The drawing under review shows one solid part. Ordinate dimensions are in mm from its lowest x, y, z. A direction names the side the tool comes from. Coordinates: 2 decimals unless noted, no trailing zeros. Write each loop counter-clockwise with the first axis right and the second up, starting at its lowest first coordinate (ties: lowest second). Pieces come first, ordered by that corner, then holes. Notation, with made-up numbers: (55.25, -1) - (114.25, -1) arc R21 cw to (114.25, 37) - close; hole circle Ø5 at (20, -20). An arc over 180 degrees is marked (long way). Put each result on its own line as item: value. Start each with the question number.
Item 1: Consider section B-B on y = 449. Give the boundary of the cut face in (x, z) (3 decimals).
Item 2: Machinability: for the marked faces 5, 6 and 7, which of the approach directions +Z, -Z, +X, -X, +Y, -Y give a long, thin tool a straight path to every point of the face, cutting with its end or side? Answer none if there is none.
Item 3: Consider section A-A on x = 92.5. Give the boundary of the cut face in (y, z).
Item 4: Mouldability with a two-part tool opening along Z and no side actions: class the marked faces 1, 2, 3 and 4 as pulls with the +Z half, pulls with the -Z half, needs draft (parallel to the pull), parting line crosses it, or undercut.
Item 5: Consider section C-C on z = 137. Give the boundary of the cut face in (x, y), then the cut area to 3 significant figures.
Item 6: For pin 1 (10 mm diameter, centred on y = 324, z = 345.5, fed in from -X); pin 2 (2 mm diameter, centred on y = 151, z = 370, fed in from +X), all flat-tipped, find the tip position at first contact; note any pin that passes through.
Item 7: To check wall thickness, follow L1, parallel to Z at x = 163, y = 318; L2, parallel to X at y = 210, z = 89.5. State the ranges of each line that lie inside material, in increasing order. Write a range as [from, to].
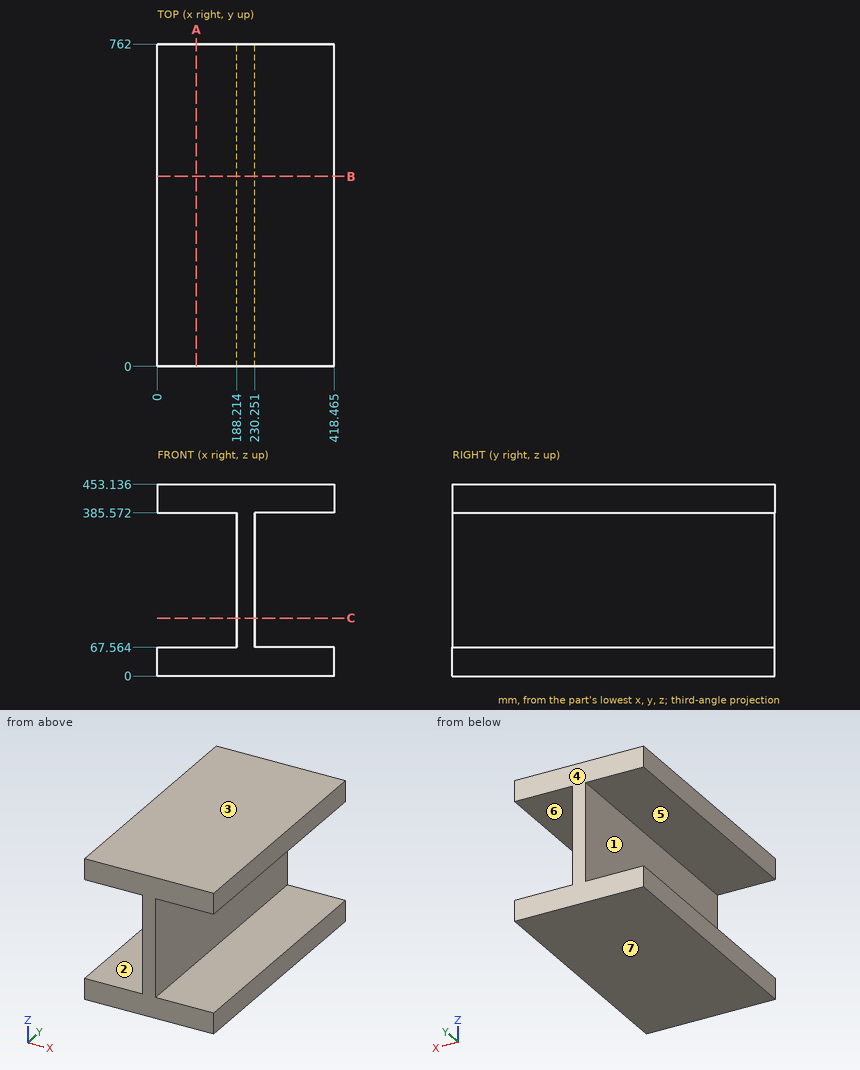
Report:
1. outline: (0, 0) - (418.465, 0) - (418.465, 67.564) - (230.251, 67.564) - (230.251, 385.572) - (418.465, 385.572) - (418.465, 453.136) - (0, 453.136) - (0, 385.572) - (188.214, 385.572) - (188.214, 67.564) - (0, 67.564) - close
2. face 5: -X, +Y, -Y
2. face 6: +X, +Y, -Y
2. face 7: -Z, +X, -X, +Y, -Y
3. outline: (0, 0) - (762, 0) - (762, 67.56) - (0, 67.56) - close; (0, 385.57) - (762, 385.57) - (762, 453.14) - (0, 453.14) - close
4. face 1: undercut
4. face 2: undercut
4. face 3: pulls with the +Z half
4. face 4: needs draft
5. outline: (188.21, 0) - (230.25, 0) - (230.25, 762) - (188.21, 762) - close
5. area: 32,000 mm²
6. pin 1: x = 188.21
6. pin 2: x = 230.25
7. L1: [0, 67.56], [385.57, 453.14]
7. L2: [188.21, 230.25]
